Autodesk Inventor part; units mm, degrees
ref_plane "YZ Plane" through (0, 0, 0) normal (1, 0, 0) x (0, 1, 0)
ref_plane "XZ Plane" through (0, 0, 0) normal (0, 1, 0) x (-1, 0, 0)
ref_plane "XY Plane" through (0, 0, 0) normal (0, 0, 1) x (1, 0, 0)
sketch "Sketch1" plane through (0, 0, 0) normal (0, 1, 0) x (-1, 0, 0)
  line L0 (35, 50) -> (-35, 50)
  line L1 (-35, 50) -> (-35, -50)
  line L2 (-35, -50) -> (35, -50)
  line L3 (35, -50) -> (35, 50)
  line L4 (35, 50) -> (-35, -50) construction
  line L5 (-35, 50) -> (35, -50) construction
  line L6 (35, 35) -> (-35, 35)
  line L7 (-35, 35) -> (-35, -35)
  line L8 (-35, -35) -> (35, -35)
  line L9 (35, -35) -> (35, 35)
  line L10 (35, 35) -> (-35, -35) construction
  line L11 (-35, 35) -> (35, -35) construction
  line L12 (0, 35) -> (0, -35)
  line L13 (35, 0) -> (-35, 0)
  line L14 (0, 0) -> (0, 15) construction
  line L15 (0, 15) -> (15, 15) construction
  line L16 (0, 0) -> (0, -15) construction
  line L17 (0, -15) -> (-15, -15) construction
  circle A0 centre (15, 15) radius 2.5
  circle A1 centre (-15, -15) radius 2.5
  dimension "d0" = 70
  dimension "d1" = 100
  dimension "d2" = 70
  dimension "d3" = 70
  dimension "d46" = 15
  dimension "d47" = 15
  dimension "d48" = 15
  dimension "d49" = 5
  dimension "d50" = 5
extrude "Extrusion1" add sketch "Sketch1" along normal blind 12 contours L3 L6 L1 L0 | L13 L12 L8 L1 | L3 L2 L1 L8 | A1
extrude "Extrusion2" add sketch "Sketch1" along normal blind 17 contours L6 L12 L13 L1
extrude "Extrusion3" add sketch "Sketch1" along normal blind 22 contours L3 L8 L12 L13
extrude "Extrusion4" add sketch "Sketch1" along normal blind 27 contours L3 L13 L12 L6 | A0
sketch "Sketch2" plane through (0, 27, 0) normal (0, 1, 0) x (1, 0, 0)
  line L0 (35, -35) -> (-35, -35) construction
  line L1 (35, 0) -> (0, 0) construction
  line L2 (-35, -35) -> (0, -35) construction
  line L3 (0, -35) -> (0, 0) construction
  line L4 (0, 0) -> (-35, 0) construction
  line L5 (-35, 0) -> (-35, -35) construction
  line L6 (0, -35) -> (-35, 0) construction
  line L7 (0, 0) -> (-35, -35) construction
  line L8 (-5, -32.5) -> (-15, -32.5)
  line L9 (-32.5, -15) -> (-32.5, -5)
  line L10 (-30, -2.5) -> (-20, -2.5)
  line L11 (-2.5, -20) -> (-2.5, -30)
  line L12 (-2.5, -32.5) -> (-32.5, -2.5) construction
  line L13 (-32.5, -32.5) -> (-2.5, -2.5) construction
  line L14 (-15, -27.5) -> (-10, -27.5)
  line L15 (-7.5, -25) -> (-7.5, -20)
  line L16 (-20, -7.5) -> (-25, -7.5)
  line L17 (-27.5, -10) -> (-27.5, -15)
  line L18 (-27.5, -27.5) -> (-7.5, -7.5) construction
  line L19 (-7.5, -27.5) -> (-27.5, -7.5) construction
  line L20 (-5, -17.5) -> (-5, -17.5)
  line L21 (-17.5, -30) -> (-17.5, -30)
  line L22 (-30, -17.5) -> (-30, -17.5)
  line L23 (-17.5, -5) -> (-17.5, -5)
  arc A0 (-17.5, -30) -> (-15, -32.5) centre (-15, -30) ccw
  arc A1 (-15, -27.5) -> (-17.5, -30) centre (-15, -30) ccw
  arc A2 (-5, -17.5) -> (-7.5, -20) centre (-5, -20) ccw
  arc A3 (-2.5, -20) -> (-5, -17.5) centre (-5, -20) ccw
  arc A4 (-5, -32.5) -> (-2.5, -30) centre (-5, -30) ccw
  arc A5 (-32.5, -15) -> (-30, -17.5) centre (-30, -15) ccw
  arc A6 (-30, -17.5) -> (-27.5, -15) centre (-30, -15) ccw
  arc A7 (-20, -7.5) -> (-17.5, -5) centre (-20, -5) ccw
  arc A8 (-17.5, -5) -> (-20, -2.5) centre (-20, -5) ccw
  arc A9 (-30, -2.5) -> (-32.5, -5) centre (-30, -5) ccw
  line L24 (5, -32.5) -> (15, -32.5)
  line L25 (32.5, -15) -> (32.5, -5)
  line L26 (30, -2.5) -> (20, -2.5)
  line L27 (2.5, -20) -> (2.5, -30)
  line L28 (15, -27.5) -> (10, -27.5)
  line L29 (7.5, -25) -> (7.5, -20)
  line L30 (20, -7.5) -> (25, -7.5)
  line L31 (27.5, -10) -> (27.5, -15)
  arc A10 (15, -32.5) -> (17.5, -30) centre (15, -30) ccw
  arc A11 (17.5, -30) -> (15, -27.5) centre (15, -30) ccw
  arc A12 (7.5, -20) -> (5, -17.5) centre (5, -20) ccw
  arc A13 (5, -17.5) -> (2.5, -20) centre (5, -20) ccw
  arc A14 (2.5, -30) -> (5, -32.5) centre (5, -30) ccw
  arc A15 (30, -17.5) -> (32.5, -15) centre (30, -15) ccw
  arc A16 (27.5, -15) -> (30, -17.5) centre (30, -15) ccw
  arc A17 (17.5, -5) -> (20, -7.5) centre (20, -5) ccw
  arc A18 (20, -2.5) -> (17.5, -5) centre (20, -5) ccw
  arc A19 (32.5, -5) -> (30, -2.5) centre (30, -5) ccw
  line L32 (7.5, 25) -> (7.5, 20)
  arc A20 (10, 27.5) -> (7.5, 25) centre (10, 25) ccw
  line L33 (15, 27.5) -> (10, 27.5)
  arc A21 (15, 27.5) -> (17.5, 30) centre (15, 30) ccw
  arc A22 (17.5, 30) -> (15, 32.5) centre (15, 30) ccw
  line L34 (5, 32.5) -> (15, 32.5)
  arc A23 (5, 32.5) -> (2.5, 30) centre (5, 30) ccw
  line L35 (2.5, 20) -> (2.5, 30)
  arc A24 (2.5, 20) -> (5, 17.5) centre (5, 20) ccw
  arc A25 (5, 17.5) -> (7.5, 20) centre (5, 20) ccw
  line L36 (-32.5, 15) -> (-32.5, 5)
  line L37 (-30, 2.5) -> (-20, 2.5)
  line L38 (-20, 7.5) -> (-25, 7.5)
  line L39 (-27.5, 10) -> (-27.5, 15)
  arc A26 (-30, 17.5) -> (-32.5, 15) centre (-30, 15) ccw
  arc A27 (-27.5, 15) -> (-30, 17.5) centre (-30, 15) ccw
  arc A28 (-27.5, 10) -> (-25, 7.5) centre (-25, 10) ccw
  arc A29 (-17.5, 5) -> (-20, 7.5) centre (-20, 5) ccw
  arc A30 (-20, 2.5) -> (-17.5, 5) centre (-20, 5) ccw
  arc A31 (-32.5, 5) -> (-30, 2.5) centre (-30, 5) ccw
  line L40 (-35, 50) -> (-35, 35) construction
  line L41 (35, -35) -> (35, 0) construction
  line L42 (-35, 35) -> (35, -35) construction
  line L43 (-10, -27.5) -> (-7.5, -27.5)
  line L44 (-7.5, -25) -> (-7.5, -27.5)
  line L45 (-27.5, -10) -> (-27.5, -7.5)
  line L46 (-27.5, -7.5) -> (-25, -7.5)
  line L47 (10, -27.5) -> (7.5, -27.5)
  line L48 (7.5, -27.5) -> (7.5, -25)
  line L49 (25, -7.5) -> (27.5, -7.5)
  line L50 (27.5, -7.5) -> (27.5, -10)
  point P0 (-17.5, -17.5)
  point P1 (-17.5, -17.5)
  point P2 (-7.5, -17.5)
  point P3 (-17.5, -27.5)
  point P4 (-17.5, -32.5)
  dimension "d12" = 30
  dimension "d13" = 30
  dimension "d16" = 15
  dimension "d17" = 5
  dimension "d18" = 10
  dimension "d19" = 10
  dimension "d20" = 2.5
fillet "Fillet1" radius 2.5 1 edges at (0, 14.5, 0)
extrude "Extrusion5" cut sketch "Sketch2" against normal blind 2.5 contours L8 A0 A1 L14 L43 L44 L15 A2 A3 L11 A4 | L9 A9 L10 A8 A7 L16 L46 L45 L17 A6 A5
extrude "Extrusion6" cut sketch "Sketch2" against normal blind 12.5 contours A14 L27 A13 A12 L29 L48 L47 L28 A11 A10 L24 | A15 A16 L31 L50 L49 L30 A17 A18 L26 A19 L25
sketch "Sketch3" plane through (0, 22, 0) normal (0, 1, 0) x (1, 0, 0)
  line L0 (0, 0) -> (0, 35) construction
  line L1 (-35, 50) -> (-35, -50) construction
  line L2 (0, 35) -> (-35, 35) construction
  line L3 (-35, 35) -> (-35, 0) construction
  line L4 (-35, 0) -> (0, 0) construction
  line L5 (0, 0) -> (0, 35) construction
  line L6 (-35, 35) -> (0, 0) construction
  line L7 (0, 35) -> (-35, 0) construction
  line L8 (-32.5, 15) -> (-32.5, 5)
  line L9 (-30, 2.5) -> (-5, 2.5)
  line L10 (-2.5, 5) -> (-2.5, 15)
  line L11 (-2.5, 32.5) -> (-32.5, 2.5) construction
  line L12 (-32.5, 32.5) -> (-2.5, 2.5) construction
  line L13 (-25, 7.5) -> (-10, 7.5)
  line L14 (-7.5, 10) -> (-7.5, 15)
  line L15 (-27.5, 15) -> (-27.5, 10)
  line L16 (-27.5, 7.5) -> (-7.5, 27.5) construction
  line L17 (-7.5, 7.5) -> (-27.5, 27.5) construction
  line L18 (-30, 17.5) -> (-30, 17.5)
  line L19 (-5, 17.5) -> (-5, 17.5)
  arc A0 (-30, 17.5) -> (-32.5, 15) centre (-30, 15) ccw
  arc A1 (-27.5, 15) -> (-30, 17.5) centre (-30, 15) ccw
  arc A2 (-5, 17.5) -> (-7.5, 15) centre (-5, 15) ccw
  arc A3 (-2.5, 15) -> (-5, 17.5) centre (-5, 15) ccw
  arc A4 (-5, 2.5) -> (-2.5, 5) centre (-5, 5) ccw
  arc A5 (-32.5, 5) -> (-30, 2.5) centre (-30, 5) ccw
  line L20 (35, 35) -> (0, 0) construction
  line L21 (0, 35) -> (35, 0) construction
  line L22 (32.5, 15) -> (32.5, 5)
  line L23 (30, 2.5) -> (5, 2.5)
  line L24 (2.5, 5) -> (2.5, 15)
  line L25 (2.5, 32.5) -> (32.5, 2.5) construction
  line L26 (32.5, 32.5) -> (2.5, 2.5) construction
  line L27 (25, 7.5) -> (10, 7.5)
  line L28 (7.5, 10) -> (7.5, 15)
  line L29 (27.5, 15) -> (27.5, 10)
  line L30 (27.5, 7.5) -> (7.5, 27.5) construction
  line L31 (7.5, 7.5) -> (27.5, 27.5) construction
  line L32 (30, 17.5) -> (30, 17.5)
  line L33 (5, 17.5) -> (5, 17.5)
  arc A6 (32.5, 15) -> (30, 17.5) centre (30, 15) ccw
  arc A7 (30, 17.5) -> (27.5, 15) centre (30, 15) ccw
  arc A8 (7.5, 15) -> (5, 17.5) centre (5, 15) ccw
  arc A9 (5, 17.5) -> (2.5, 15) centre (5, 15) ccw
  arc A10 (2.5, 5) -> (5, 2.5) centre (5, 5) ccw
  arc A11 (30, 2.5) -> (32.5, 5) centre (30, 5) ccw
  arc A12 (25, 7.5) -> (27.5, 10) centre (25, 10) ccw
  arc A13 (7.5, 10) -> (10, 7.5) centre (10, 10) ccw
  line L34 (0, 17.5) -> (35, 17.5) construction
  line L35 (35, 0) -> (35, 50) construction
  line L36 (2.5, 30) -> (2.5, 20)
  line L37 (27.5, 20) -> (27.5, 25)
  line L38 (35, 0) -> (0, 35) construction
  line L39 (25, 27.5) -> (10, 27.5)
  line L40 (30, 32.5) -> (5, 32.5)
  arc A14 (32.5, 30) -> (30, 32.5) centre (30, 30) ccw
  line L41 (32.5, 20) -> (32.5, 30)
  arc A15 (27.5, 20) -> (30, 17.5) centre (30, 20) ccw
  arc A16 (30, 17.5) -> (32.5, 20) centre (30, 20) ccw
  line L42 (7.5, 25) -> (7.5, 20)
  arc A17 (5, 32.5) -> (2.5, 30) centre (5, 30) ccw
  arc A18 (5, 17.5) -> (7.5, 20) centre (5, 20) ccw
  arc A19 (2.5, 20) -> (5, 17.5) centre (5, 20) ccw
  line L43 (-27.5, 10) -> (-27.5, 7.5)
  line L44 (-27.5, 7.5) -> (-25, 7.5)
  line L45 (-10, 7.5) -> (-7.5, 7.5)
  line L46 (-7.5, 7.5) -> (-7.5, 10)
  line L47 (7.5, 25) -> (7.5, 27.5)
  line L48 (7.5, 27.5) -> (10, 27.5)
  line L49 (25, 27.5) -> (27.5, 27.5)
  line L50 (27.5, 27.5) -> (27.5, 25)
  point P0 (-17.5, 17.5)
  point P1 (17.5, 17.5)
  dimension "d26" = 30
  dimension "d30" = 2.5
extrude "Extrusion7" cut sketch "Sketch3" against normal blind 2.5 contours A0 A1 L15 L43 L44 L13 L45 L46 L14 A2 A3 L10 A4 L9 A5 L8
extrude "Extrusion8" cut sketch "Sketch3" against normal blind 12.5 contours A15 L37 L50 L49 L39 L48 L47 L42 A18 A19 L36 A17 L40 A14 L41 A16
sketch "Sketch5" plane through (0, 12, 0) normal (0, 1, 0) x (1, 0, 0)
  line L0 (-35, -50) -> (35, -50) construction
  line L1 (-35, -50) -> (-35, -42.5) construction
  line L2 (-35, 50) -> (-35, -50) construction
  line L3 (-35, -42.5) -> (34.9391, -42.5) construction
  line L4 (-35, 50) -> (-35, 35) construction
  line L5 (-35, 42.5) -> (35, 42.5) construction
  line L6 (35, 0) -> (35, 50) construction
  line L7 (0, 42.5) -> (-25, 42.5) construction
  line L8 (-25, 42.5) -> (25, 42.5) construction
  line L9 (25, 42.5) -> (25, -42.5) construction
  line L10 (25, -42.5) -> (-25, -42.5) construction
  point P0 (0, 0)
  dimension "d35" = 7.5
  dimension "d36" = 25
  dimension "d37" = 50
  dimension "d38" = 50
hole "Hole1" at (-25, 12, 42.5) at (-25, 12, -42.5) at (25, 12, -42.5) at (25, 12, 42.5) direction (0, -1, 0) diameter 6.1 end through all countersink diameter 11 countersink angle 90
sketch "Sketch6" plane through (0, 27, 0) normal (0, 1, 0) x (1, 0, 0)
  line L0 (-35, 0) -> (0, 0)
  arc A0 (-10, 0) -> (0, -10) centre (0, 0) ccw
  line L1 (0, -10) -> (0, 0)
  line L2 (-10, 0) -> (0, 0)
  dimension "d54" = 10
extrude "Extrusion10" add sketch "Sketch6" along normal blind 5
sketch "Sketch7" plane through (0, 0, 0) normal (0, -1, 0) x (1, 0, 0)
  circle A0 centre (25, -42.5) radius 3.05 construction
  line L0 (-25, 42.5) -> (25, 42.5) construction
  line L1 (25, 42.5) -> (25, -42.5) construction
  line L2 (25, -42.5) -> (-25, -42.5) construction
  line L3 (-25, -42.5) -> (-25, 42.5) construction
  line L4 (-25, 42.5) -> (25, -42.5) construction
  line L5 (25, 42.5) -> (-25, -42.5) construction
  point P0 (0, 0)
extrude "Extrusion11" cut sketch "Sketch1" along normal blind 11 contours A0 | A1
properties part number "SmallTool20mm"
Build history of the part. All positions in model axes, mm. A direction names the side the tool comes from. Round coordinates to 2 decimals unless told otherwise and drop trailing zeros. Write each loop counter-clockwise with the first axis right and the second up, starting at its lowest first coordinate (ties: lowest second). Pieces come first, ordered by that corner, then holes. Notation, with made-up numbers: (30.5, 11) - (80.5, 11) arc R26 cw to (80.5, 46) - close; hole circle Ø5 at (-17, -6.5). An arc over 180 degrees is marked (long way). Answer as CSV lines item,"result".
Q1. Cut at A-A (x = -25). State how many separate pieces and enclosed holes the cut face has, and give its area (3 significant figures).
Report:
separate pieces,"3"
enclosed holes,"0"
area,"1,890 mm^2"
Q2. Drop flat-ended pins along their axis: pin 1 (4.5 mm diameter, centred on x = 12.5, z = 28, fed in from +Y); pin 2 (4 mm diameter, centred on x = -6, y = 25.5, fed in from -Z); pin 3 (4.5 mm diameter, centred on x = -25, z = 9, fed in from +Y); pin 4 (5 mm diameter, centred on x = 25, z = 42.5, fed in from +Y). Give the stop position or say it passes through.
Report:
pin 1,"stops at y = 17"
pin 2,"stops at z = 0"
pin 3,"stops at y = 27"
pin 4,"passes through"
Q3. Cut at C-C (z = 24.5). Write the cut outline in (x, y), and give its area (4 significant figures).
Report:
outline,"(-35, 0) - (35, 0) - (35, 17) - (7.5, 17) - (7.5, 14.5) - (2.5, 14.5) - (2.5, 17) - (0, 17) - (0, 27) - (-2.5, 27) - (-2.5, 24.5) - (-7.5, 24.5) - (-7.5, 27) - (-35, 27) - close"
area,"1,515 mm^2"
Q4. Tool access for faces 5 (the cylindrical face through (-12.5, 5.4, 14.9)), 6 (the cylindrical face through (-4.9, 20.8, -17.5)), 7 (the flat face through (0, 20, 0)): list every direction of +Z, -Z, +X, -X, +Y, -Y with a clear straight run to the whole face (end or side of a thin tool).
Report:
face 5,"-Y"
face 6,"+Y"
face 7,"-Z, +X, +Y"
Q5. Cut at B-B (z = -22). Write the cut outline in (x, y), and give its area (4 significant figures).
Report:
outline,"(-35, 0) - (35, 0) - (35, 12) - (32.5, 12) - (32.5, 9.5) - (27.5, 9.5) - (27.5, 12) - (7.5, 12) - (7.5, 9.5) - (2.5, 9.5) - (2.5, 12) - (0, 12) - (0, 22) - (-35, 22) - close"
area,"1,165 mm^2"
Q6. Pull direction Z, two halves, no side cores. Call faces 1 (the flat face through (-18, 19.5, -7)), 2 (the flat face through (17, 11, -27.5)), 3 (the flat face through (19, 14, 0)), 4 (the flat face through (-17, 27, 18)): +Z half, -Z half, draft (parallel to the pull), parting line (faces both ways), or undercut.
Report:
face 1,"undercut"
face 2,"undercut"
face 3,"-Z half"
face 4,"draft"
Q7. Drill centre lines: probe 1 along X at (y, z) = (6.5, 42.5); probe 2 along Z at (x, y) = (-25, 6); probe 3 along Z at (x, y) = (15, 8.75). Where is each one in solid material? Low to high. Write a range as [from, to].
Report:
probe 1,"x = [-35, -28.05], [-21.95, 21.95], [28.05, 35]"
probe 2,"z = [-50, -45.55], [-39.45, 39.45], [45.55, 50]"
probe 3,"z = [-50, -17.5], [-12.5, 50]"
